```python
from build123d import *

# Parameters (mm, degrees)
CHANFREIN1_SIZE              = 0.3
CONG_1_R                     = 0.5
ESQUISSE2_R                  = 5
BOSS_EXTRU_1_DEPTH           = 2
CONG_2_R                     = 1.5
R_P_TITION_CIRCULAIRE1_COUNT = 4


with BuildPart() as part:
    # Esquisse1 → R_volution1 (revolve)
    with BuildSketch(Plane.XY, mode=Mode.PRIVATE) as r_volution1_sk:
        Polygon((0, 0), (0, 11), (2, 11), (2, 21), (82, 21), (82, 0), align=None)
    revolve(r_volution1_sk.sketch.rotate(Axis((-33.755102041, 0, 0), (1, 0, 0)), 90), axis=Axis((-33.755102041, 0, 0), (1, 0, 0)))

    # Chanfrein1
    chanfrein1_edges = [part.edges().sort_by_distance(p)[0] for p in [
        (2, 0, -21),
        (0, 0, -11),
    ]]
    chamfer(chanfrein1_edges, length=CHANFREIN1_SIZE)

    # Cong_1
    cong_1_edges = [part.edges().sort_by_distance(p)[0] for p in [
        (82, 0, -21),
    ]]
    fillet(cong_1_edges, radius=CONG_1_R)

    # Esquisse2 → Boss.-Extru.1 (add)
    with BuildSketch(Plane(origin=(82, 0, 0), x_dir=(0, 0, -1), z_dir=(1, 0, 0))):
        with Locations(Location((0, 15.5, 0), (0, 0, 90))):
            Circle(ESQUISSE2_R)
    extrude(amount=BOSS_EXTRU_1_DEPTH)

    # Cong_2
    cong_2_edges = [part.edges().sort_by_distance(p)[0] for p in [
        (84, 10.5, 0),
    ]]
    fillet(cong_2_edges, radius=CONG_2_R)

    # Esquisse4 → Trou pour taraudage pour trou taraud_ M4 (revolve, cut)
    with BuildSketch(Plane(origin=(2, 16, 0), x_dir=(0, 0, 1), z_dir=(0, 1, 0))):
        Polygon((0, 0), (0, 8.991420021), (1.65, 8), (1.65, 0), align=None)
    trou_pour_taraudage_pour_trou_taraud_m4 = revolve(axis=Axis((-4.35, 16, 0), (1, 0, 0)), mode=Mode.SUBTRACT)

    # R_p_tition circulaire1: Trou pour taraudage pour trou taraud_ M4 ×4 about axis
    r_p_tition_circulaire1_axis = Axis((0, 0, 0), (1, 0, 0))
    for i in range(1, R_P_TITION_CIRCULAIRE1_COUNT):
        add(trou_pour_taraudage_pour_trou_taraud_m4.rotate(r_p_tition_circulaire1_axis, i * 360 / R_P_TITION_CIRCULAIRE1_COUNT), mode=Mode.SUBTRACT)


solid = part.part
```
Could you check a few things on this model? Use its own coordinates, in mm. A direction names the side the tool comes from. Round coordinates to 2 decimals unless told otherwise and drop trailing zeros. Loops run counter-clockwise (first coordinate to the right, second up) from the corner with the lowest first, then second, coordinate; pieces in that order, holes last.
Q1. Please list where these lines run through material, in increasing order: L1, parallel to Y at x = 8, z = 0; L2, parallel to X at y = -7, z = 17; L3, parallel to X at y = 0, z = -16.
Q2. Thinking about a two-plate mould opening in Z: for faces 1 (the cylindrical face through (5.9, -0.4, -17.6)), 2 (the cylindrical face through (1.16, 10.74, -2.38)), 3 (the flat face through (84, 15, 0)), which applies, pulls with the +Z half, pulls with the -Z half, needs draft (parallel to the pull), parting line crosses it, or undercut?
Q3. For P1, Ø3, axis at x = 73, y = 11, coming from the +Z side; P2, Ø2.5, axis at y = 16, z = 0, coming from the -X side; P3, Ø6, axis at x = 44, z = -13.5, coming from the -Y side, each with a flat end and sliding along its axis, tell me the tip position at first contact or that it passes through.
Q4. On a 3-axis mill with a long thin cutter (end or side, diameter ignored), from which of +Z, -Z, +X, -X, +Y, -Y can I reach the whole of each face in a straight line? I mean faces 4 (the cylindrical face through (5.9, -17.6, 0.4)), 5 (the flat face through (0, 0, 0)), 6 (the cylindrical face through (82.25, 20.27, 1.5)). Say none if no direction works.
Q5. I want a section at A-A (x = 49.5). Write out the boundary of the cut face in (y, z), and give its area (3 significant figures).
Answer below:
1. L1: y = -21 to -17.65, -14.35 to 14.35, 17.65 to 21
1. L2: x = 2 to 82
1. L3: x = 10.99 to 82
2. face 1: undercut
2. face 2: parting line crosses it
2. face 3: needs draft
3. P1: stops at z = 18.73
3. P2: stops at x = 10.24
3. P3: stops at y = -18.19
4. face 4: -X
4. face 5: +Z, -Z, -X, +Y, -Y
4. face 6: +X
5. outline: circle Ø42 at (0, 0)
5. area: 1,390 mm2
